Here's how the part is built. I have some questions about the finished solid (model axes, mm). Face numbers are marked on the shaded views. A direction names the side the tool comes from. Coordinates: 2 decimals unless noted, no trailing zeros. Write each loop counter-clockwise with the first axis right and the second up, starting at its lowest first coordinate (ties: lowest second). Pieces come first, ordered by that corner, then holes. Notation, with made-up numbers: (-40, 4.5) -> (8, 4.5) arc R26 cw to (8, 29.5) -> close; hole circle Ø7 at (33.5, 39.5). An arc over 180 degrees is marked (long way). Use a Markdown table: item, result. Add a question column.
Item 1: If I drill on line 1 along Z through (x, y) = (32, -505); line 2 along Y through (x, z) = (21, -12); line 3 along X through (y, z) = (-507, 37), over which ranges is the centre line in solid material (lowest first)? Write a range as from..to.
Item 2: On a 3-axis mill with a long thin cutter (end or side, diameter ignored), from which of +Z, -Z, +X, -X, +Y, -Y can I reach the whole of each face in a straight line? I mean the marked faces 5, 6 and 7. Say none if no direction works.
Item 3: If we mould it in two halves opening along Y, with no side actions, what happens to the marked faces 1, 2, 3 and 4? For each: pulls with the +Y half, pulls with the -Y half, needs draft (parallel to the pull), parting line crosses it, or undercut.
Item 4: Imagine slicing it at B-B, the plane z = -3.5. Write out the boundary of the cut face in (x, y).
Item 5: Imagine slicing it at A-A, the plane y = -435. Write out the boundary of the cut face in (x, z).
Item 6: Will these pins go through, and if not, where does the flat tip stop? pin 1 Ø1 at (y, z) = (-383.5, -4.5) entering from +X; pin 2 Ø12.5 at (x, z) = (29.5, -6.5) entering from +Y; pin 3 Ø12.5 at (x, z) = (37, 22) entering from -Y; pin 4 Ø9.5 at (x, z) = (32.5, 37.5) entering from -Y.
Item 7: Imagine slicing it at C-C, the plane x = 8. Write out the boundary of the cut face in (y, z), and give its area (3 significant figures).
```python
from build123d import *

# Parameters (mm, degrees)
F0_W     = 40
F0_H     = 40
F1_DEPTH = 600
F2_R     = 1.5
F3_W     = 10
F3_H     = 100
F4_DEPTH = 25
F5_R     = 12.49999
F7_D     = 12
F7_DEPTH = 450
F7_TIP   = 3.6051637142


# Not quite as in the source:
# - a fillet or chamfer is up to 0.001 mm smaller than in the source, because OpenCascade refuses the exact size


with BuildPart() as f1:
    # F0 (on Front) → F1 (new body)
    with BuildSketch(Plane.XZ):
        Rectangle(F0_W, F0_H)
    extrude(amount=F1_DEPTH)

    # F2
    f2_edges = [f1.edges().sort_by_distance(p)[0] for p in [
        (-20, -300, 20),
        (-20, -300, -20),
        (20, -300, 20),
        (20, -300, -20),
    ]]
    fillet(f2_edges, radius=F2_R)

    # F3 (on face) → F4 (join)
    with BuildSketch(Plane.YZ.offset(20)):
        with Locations((-505, 0)):
            Rectangle(F3_W, F3_H)
        with Locations((-95, 0)):
            Rectangle(F3_W, F3_H)
    extrude(amount=F4_DEPTH)

    # F5 (radius 12.5 in the source; OpenCascade refuses exactly that, so slightly less here)
    f5_edges = [f1.edges().sort_by_distance(p)[0] for p in [
        (45, -505, 50),
        (20, -505, 50),
        (45, -95, 50),
        (20, -95, 50),
        (45, -95, -50),
        (45, -505, -50),
        (20, -505, -50),
        (20, -95, -50),
    ]]
    fillet(f5_edges, radius=F5_R)

    # F7
    with Locations(Plane.XZ.offset(510)):
        with Locations((32.5, 37.5), (32.5, -37.5)):
            Hole(F7_D / 2, depth=F7_DEPTH)
            with Locations((0, 0, -(F7_DEPTH + F7_TIP / 2))):  # 118° drill point
                Cone(0, F7_D / 2, F7_TIP, mode=Mode.SUBTRACT)


solid = f1.part
```
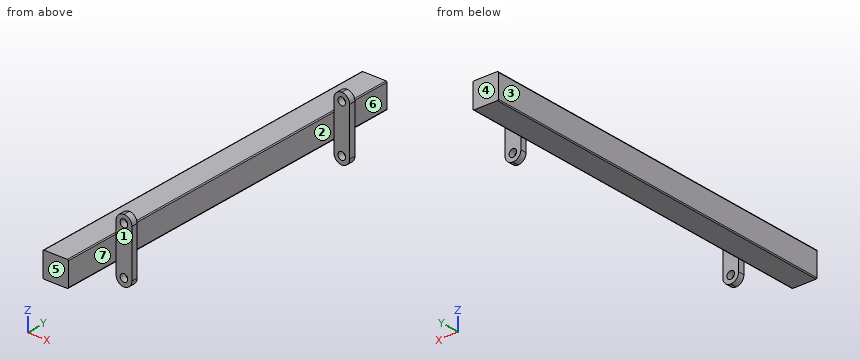
Ans:
| question | item | result |
|---|---|---|
| 1 | line 1 | z = -49.99..-43.48, -31.52..31.52, 43.48..49.99 |
| 1 | line 2 | y = -510..-500, -100..-90 |
| 1 | line 3 | x = 20..26.52, 38.48..45 |
| 2 | face 5 | +Z, -Z, +X, -X, -Y |
| 2 | face 6 | +Z, -Z, +X, +Y |
| 2 | face 7 | +Z, -Z, +X, -Y |
| 3 | face 1 | pulls with the -Y half |
| 3 | face 2 | undercut |
| 3 | face 3 | needs draft |
| 3 | face 4 | pulls with the +Y half |
| 4 | outline | (-20, -600) -> (20, -600) -> (20, -510) -> (45, -510) -> (45, -500) -> (20, -500) -> (20, -100) -> (45, -100) -> (45, -90) -> (20, -90) -> (20, 0) -> (-20, 0) -> close |
| 5 | outline | (-20, -18.5) arc R1.5 ccw to (-18.5, -20) -> (18.5, -20) arc R1.5 ccw to (20, -18.5) -> (20, 18.5) arc R1.5 ccw to (18.5, 20) -> (-18.5, 20) arc R1.5 ccw to (-20, 18.5) -> close |
| 6 | pin 1 | stops at x = 20 |
| 6 | pin 2 | stops at y = -90 |
| 6 | pin 3 | stops at y = -510 |
| 6 | pin 4 | passes through |
| 7 | outline | (-600, -20) -> (0, -20) -> (0, 20) -> (-600, 20) -> close |
| 7 | area | 24,000 mm^2 |
